Could you check a few things on this drawing? It's one solid part, dimensions in mm from its lowest x, y, z. A direction names the side the tool comes from. Round coordinates to 2 decimals unless told otherwise and drop trailing zeros. Write each loop counter-clockwise with the first axis right and the second up, starting at its lowest first coordinate (ties: lowest second). Pieces come first, ordered by that corner, then holes. Notation, with made-up numbers: (57, -9) - (91, -9) arc R23 cw to (91, 9) - close; hole circle Ø7 at (26.5, 58). An arc over 180 degrees is marked (long way). Write item = value, one per line. Start each with the question number.
Item 1: If we section it at D-D (y = 6): Please give me the cut outline in (x, z).
Item 2: If I drill on line 1 along Z through (x, y) = (30, 14.5); line 2 along Z through (x, y) = (14, 25.5); line 3 along X through (y, z) = (25.5, 5) (3 decimals), over which ranges is the centre line in solid material (lowest first)? Write a range as [from, to].
Item 3: If we section it at C-C (z = 5.5): Please give me the cut outline in (x, y) (3 decimals), and give its area (3 significant figures).
Item 4: Which directions (+Z, -Z, +X, -X, +Y, -Y) give clear straight access to the entire face, cutting with the end or side of a thin tool? Please do the marked faces 4, 5 and 6.
Item 5: If we section it at A-A (y = 19.05): Please give me the cut outline in (x, z) (1 decimal), and give its area (3 significant figures).
Item 6: Thinking about a two-plate mould opening in X: for the marked faces 1, 2 and 3, which applies, pulls with the +X half, pulls with the -X half, needs draft (parallel to the pull), parting line crosses it, or undercut?
Item 7: For P1, Ø6, axis at x = 23, z = 3.5, coming from the +Y side; P2, Ø5, axis at x = 28, z = 22.5, coming from the -Y side; P3, Ø5, axis at x = 12, z = 7.5, coming from the -Y side (3 decimals); P4, Ø2.5, axis at y = 19.5, z = 7, coming from the +X side (3 decimals), each with a flat end and sliding along its axis, tell me the tip position at first contact or that it passes through.
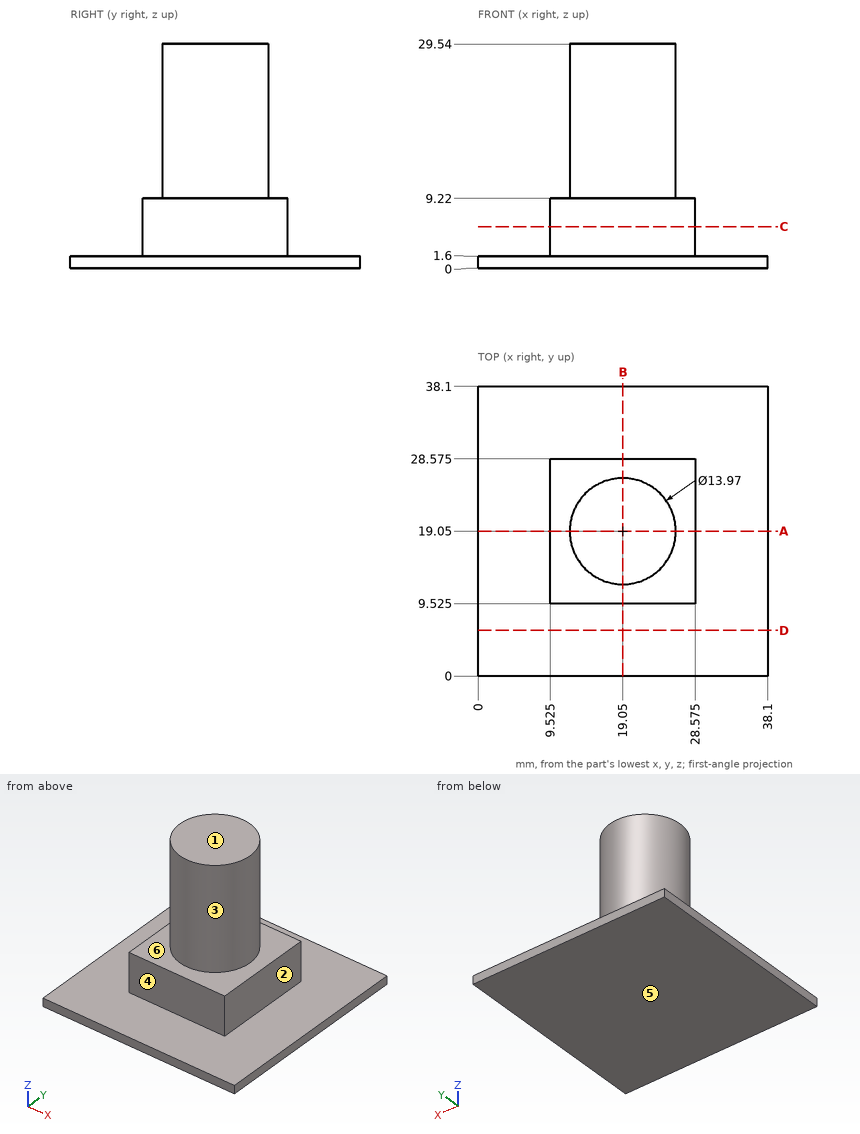
Reply:
q1.outline = (0, 0) - (38.1, 0) - (38.1, 1.6) - (0, 1.6) - close
q2.line_1 = [0, 1.6]
q2.line_2 = [0, 9.22]
q2.line_3 = [9.525, 28.575]
q3.outline = (9.525, 9.525) - (28.575, 9.525) - (28.575, 28.575) - (9.525, 28.575) - close
q3.area = 363 mm2
q4.face_4 = +Z, +X, -X, -Y
q4.face_5 = -Z, +X, -X, +Y, -Y
q4.face_6 = +Z
q5.outline = (0, 0) - (38.1, 0) - (38.1, 1.6) - (28.6, 1.6) - (28.6, 9.2) - (26, 9.2) - (26, 29.5) - (12.1, 29.5) - (12.1, 9.2) - (9.5, 9.2) - (9.5, 1.6) - (0, 1.6) - close
q5.area = 490 mm2
q6.face_1 = needs draft
q6.face_2 = pulls with the +X half
q6.face_3 = parting line crosses it
q7.P1 = 38.1
q7.P2 = 16.37
q7.P3 = 9.525
q7.P4 = 28.575
